Work out the finished part from the listing and answer in its coordinate system (mm). Round coordinates to 2 decimals unless told otherwise and drop trailing zeros. Write each loop counter-clockwise with the first axis right and the second up, starting at its lowest first coordinate (ties: lowest second). Pieces come first, ordered by that corner, then holes. Notation, with made-up numbers: M 22,-36.5 L 73,-36.5 A5 cw 73,-30.5 Z; hole C 31,64 d8. An arc over 180 degrees is marked long. Answer in a Markdown table with one row per item.
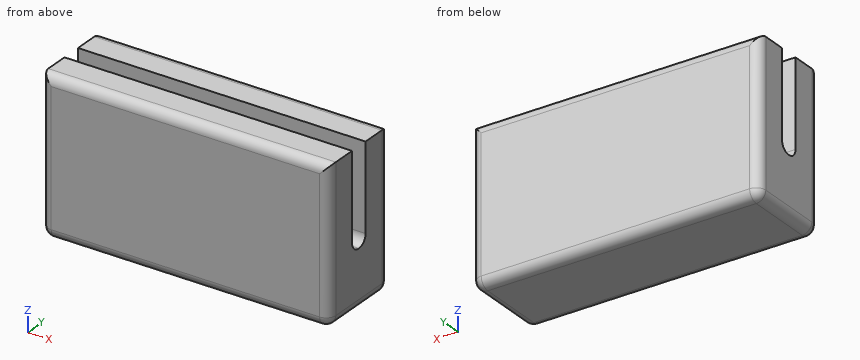
```python
from build123d import *

# Parameters (mm, degrees)
F0_W     = 30
F0_H     = 9
F1_DEPTH = 16
F2_W     = 30
F2_H     = 2.056142
F3_DEPTH = 10
F4_R     = 1
F5_R     = 1


with BuildPart() as f1:
    # F0 (on Top) → F1 (new body)
    with BuildSketch(Plane.XY):
        Rectangle(F0_W, F0_H)
    extrude(amount=F1_DEPTH)

    # F2 (on face) → F3 (cut)
    with BuildSketch(Plane.XY.offset(16)):
        Rectangle(F2_W, F2_H)
    extrude(amount=-F3_DEPTH, mode=Mode.SUBTRACT)

    # F4
    f4_edges = [f1.edges().sort_by_distance(p)[0] for p in [
        (0, -1.028071, 6),
        (0, 1.028071, 6),
    ]]
    fillet(f4_edges, radius=F4_R)

    # F5
    f5_edges = [f1.edges().sort_by_distance(p)[0] for p in [
        (0, 4.5, 16),
        (0, -4.5, 16),
        (0, 4.5, 0),
        (0, -4.5, 0),
        (15, 0, 0),
        (15, -4.5, 8),
        (15, 4.5, 8),
        (-15, 4.5, 8),
        (-15, 0, 0),
        (-15, -4.5, 8),
    ]]
    fillet(f5_edges, radius=F5_R)


solid = f1.part
```
1. The part is cut by section C-C (y = 0.5). Determine the outline of the cut face in (x, z), plus the area to 3 significant figures.
Calculated:
| item | result |
|---|---|
| outline | M -15,1 A1 ccw -14,0 L 14,0 A1 ccw 15,1 L 15,6.12 L -15,6.12 Z |
| area | 183 mm² |
2. The part is cut by section A-A (z = 9). Determine the outline of the cut face in (x, y), plus the area to 3 significant figures.
Calculated:
| item | result |
|---|---|
| outline | M -15,-3.5 A1 ccw -14,-4.5 L 14,-4.5 A1 ccw 15,-3.5 L 15,-1.03 L -15,-1.03 Z; M -15,1.03 L 15,1.03 L 15,3.5 A1 ccw 14,4.5 L -14,4.5 A1 ccw -15,3.5 Z |
| area | 207 mm² |
3. Consider line 1 along Y through (x, z) = (8, 14.75); line 2 along Z through (x, y) = (3.5, 0); line 3 along Z through (x, y) = (-7, 0.5). Determine where each line is inside the solid, lowest interval first. Write a range as from..to.
Calculated:
| item | result |
|---|---|
| line 1 | y = -4.5..-1.03, 1.03..4.5 |
| line 2 | z = 0..6 |
| line 3 | z = 0..6.12 |
4. The part is cut by section B-B (x = 9.5). Determine the outline of the cut face in (y, z).
Calculated:
| item | result |
|---|---|
| outline | M -4.5,1 A1 ccw -3.5,0 L 3.5,0 A1 ccw 4.5,1 L 4.5,15 A1 ccw 3.5,16 L 1.03,16 L 1.03,7 A1 cw 0.03,6 L -0.03,6 A1 cw -1.03,7 L -1.03,16 L -3.5,16 A1 ccw -4.5,15 Z |
5. Given pin 1 (1.5 mm diameter, centred on x = 7.5, y = 0, fed in from +Z), flat-ended and moving along its own axis, determine where the tip first touches the part or whether it passes through.
Calculated:
| item | result |
|---|---|
| pin 1 | stops at z = 6.31 |
